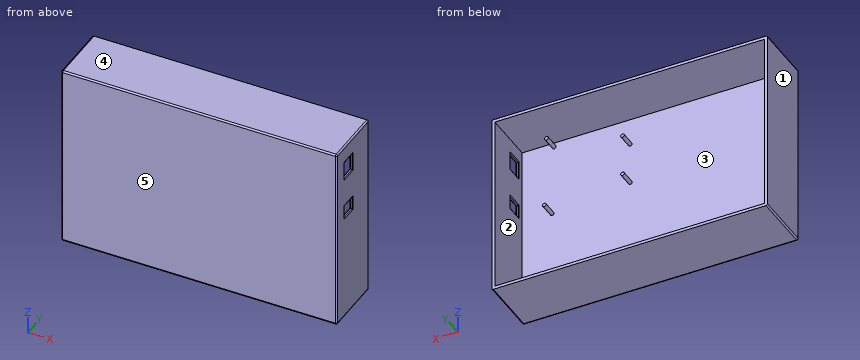
```python
from build123d import *

# Parameters (mm, degrees)
IZIM2_W                     = 184
IZIM2_H                     = 124
Y_KSEKLIK_EKSTR_ZYON1_DEPTH = 40
IZIM3_W                     = 180
IZIM3_H                     = 120
KES_EKSTR_ZYON1_DEPTH       = 35
KES_EKSTR_ZYON3_DEPTH       = 100
KES_EKSTR_ZYON3_DEPTH_BACK  = 57
IZIM9_W                     = 12
IZIM9_H                     = 11
IZIM9_W_2                   = 9
IZIM10_R                    = 1.225
Y_KSEKLIK_EKSTR_ZYON2_DEPTH = 10
RADYUS1_R                   = 1
RADYUS2_R                   = 0.5


with BuildPart() as part:
    # Çizim2 → Yükseklik-Ekstrüzyon1 (new body)
    with BuildSketch(Plane(origin=(0, 0, 0), x_dir=(1, 0, 0), z_dir=(0, 1, 0))):
        Rectangle(IZIM2_W, IZIM2_H)
    extrude(amount=Y_KSEKLIK_EKSTR_ZYON1_DEPTH)

    # Çizim3 → Kes-Ekstrüzyon1 (cut)
    with BuildSketch(Plane(origin=(0, 40, 0), x_dir=(1, 0, 0), z_dir=(0, 1, 0))):
        Rectangle(IZIM3_W, IZIM3_H)
    extrude(amount=-KES_EKSTR_ZYON1_DEPTH, mode=Mode.SUBTRACT)

    # Çizim9 → Kes-Ekstrüzyon3 (cut, two sides: drawn at the far end of the back side and taken through both)
    with BuildSketch(Plane(origin=(92, 0, 0), x_dir=(0, 0, -1), z_dir=(1, 0, 0)).offset(-KES_EKSTR_ZYON3_DEPTH_BACK)):
        with Locations((-44.5, 14.8)):
            Rectangle(IZIM9_W, IZIM9_H)
        with Locations((-14.35, 14.8)):
            Rectangle(IZIM9_W_2, IZIM9_H)
    extrude(amount=KES_EKSTR_ZYON3_DEPTH + KES_EKSTR_ZYON3_DEPTH_BACK, mode=Mode.SUBTRACT)

    # Çizim10 → Yükseklik-Ekstrüzyon2 (add)
    with BuildSketch(Plane(origin=(0, 5, 0), x_dir=(1, 0, 0), z_dir=(0, 1, 0))):
        with Locations(Location((70, -8.75, 0), (0, 0, 90))):
            Circle(IZIM10_R)
        with Locations(Location((68.6, -57.05, 0), (0, 0, 90))):
            Circle(IZIM10_R)
        with Locations(Location((17.84, -41.9, 0), (0, 0, 90))):
            Circle(IZIM10_R)
        with Locations(Location((17.81, -13.95, 0), (0, 0, 90))):
            Circle(IZIM10_R)
    extrude(amount=Y_KSEKLIK_EKSTR_ZYON2_DEPTH)

    # Radyus1
    radyus1_edges = [part.edges().sort_by_distance(p)[0] for p in [
        (-92, 0, 0),
        (0, 0, 62),
        (92, 0, 0),
        (0, 0, -62),
        (-92, 20, -62),
        (-92, 20, 62),
        (92, 20, 62),
        (92, 20, -62),
    ]]
    fillet(radyus1_edges, radius=RADYUS1_R)

    # Radyus2
    radyus2_edges = [part.edges().sort_by_distance(p)[0] for p in [
        (90, 20.3, 44.5),
        (90, 14.8, 38.5),
        (90, 9.3, 44.5),
        (90, 14.8, 50.5),
        (90, 20.3, 14.35),
        (90, 14.8, 9.85),
        (90, 9.3, 14.35),
        (90, 14.8, 18.85),
        (92, 14.8, 18.85),
        (92, 9.3, 14.35),
        (92, 14.8, 9.85),
        (92, 20.3, 14.35),
        (92, 14.8, 50.5),
        (92, 9.3, 44.5),
        (92, 14.8, 38.5),
        (92, 20.3, 44.5),
    ]]
    fillet(radyus2_edges, radius=RADYUS2_R)


solid = part.part
```
Design review of the part built by this model. Coordinates are the model's own, in mm. Face numbers are marked on the shaded views. A direction names the side the tool comes from. Give positions to 0.01 mm unless a question says otherwise; leave off trailing zeros. Write each loop counter-clockwise with the first axis right and the second up, starting at its lowest first coordinate (ties: lowest second). Pieces come first, ordered by that corner, then holes. Notation, with made-up numbers: (-22.5, -38.75) - (-9.5, -38.75) arc R14 ccw to (-9.5, -26.75) - close; hole circle Ø6 at (48.25, 86). An arc over 180 degrees is marked (long way). Return JSON: item names as keys, results as strings. Group by question number.
(1) We need section B-B, the plane y = 27. Give the boundary of the cut face in (x, z), then the cut area to 3 significant figures.
(2) Insertion check: pin 1 (1.2 mm diameter, centred on x = 68.5, z = 57.5, fed in from +Y); pin 2 (3 mm diameter, centred on x = 21.5, z = -26, fed in from +Y). Each pin has a flat end and moves straight along its axis. Give the tip position at first contact, or say it passes through.
(3) We need section C-C, the plane x = -52. Give the boundary of the cut face in (y, z).
(4) Machinability: for the marked faces 1 and 2, which of the approach directions +Z, -Z, +X, -X, +Y, -Y give a long, thin tool a straight path to every point of the face, cutting with its end or side? Answer none if there is none.
(5) Mouldability with a two-part tool opening along Z and no side actions: class the marked faces 3, 4 and 5 as +Z half, -Z half, draft (parallel to the pull), parting line (faces both ways), or undercut.
(6) To check wall thickness, follow probe 1 along Z at (x, y) = (-78.5, 13); probe 2 along X at (y, z) = (29.5, -5); probe 3 along Y at (x, z) = (-56.5, -27.5). State the ranges of each line that lie inside material, in increasing order.
(7) We need section A-A, the plane z = -30. Give the boundary of the cut face in (x, y).
Reported:
{
 "1": {"outline": "(-92, -61) arc R1 ccw to (-91, -62) - (91, -62) arc R1 ccw to (92, -61) - (92, 61) arc R1 ccw to (91, 62) - (-91, 62) arc R1 ccw to (-92, 61) - close; hole (-90, -60) - (90, -60) - (90, 60) - (-90, 60) - close", "area": "1,220 mm2"},
 "2": {"pin 1": "stops at y = 15", "pin 2": "stops at y = 5"},
 "3": {"outline": "(0, -61) arc R1 ccw to (1, -62) - (40, -62) - (40, -60) - (5, -60) - (5, 60) - (40, 60) - (40, 62) - (1, 62) arc R1 ccw to (0, 61) - close"},
 "4": {"face 1": "+Z, -Z, -X, +Y, -Y", "face 2": "+Y"},
 "5": {"face 3": "undercut", "face 4": "+Z half", "face 5": "draft"},
 "6": {"probe 1": "z = -62 to -60, 60 to 62", "probe 2": "x = -92 to -90, 90 to 92", "probe 3": "y = 0 to 5"},
 "7": {"outline": "(-92, 1) arc R1 ccw to (-91, 0) - (91, 0) arc R1 ccw to (92, 1) - (92, 40) - (90, 40) - (90, 5) - (-90, 5) - (-90, 40) - (-92, 40) - close"}
}
